CAD build for the part. Positions are in the model's coordinates, mm. Round coordinates to 2 decimals unless told otherwise and drop trailing zeros. Loops run counter-clockwise (first coordinate to the right, second up) from the corner with the lowest first, then second, coordinate; pieces in that order, holes last.
```python
from build123d import *

# Parameters (mm, degrees)
F0_W     = 101.6
F0_H     = 6.096
F1_DEPTH = 101.6
F2_W     = 6.35
F2_H     = 50.8
F2_H_2   = 25.4
F3_DEPTH = 25.4
F4_R     = 2.032


with BuildPart() as f1:
    # F0 (on Front) → F1 (new body)
    with BuildSketch(Plane.XZ):
        with Locations((2.470545, 16.174641)):
            Rectangle(F0_W, F0_H)
    extrude(amount=F1_DEPTH)

    # F2 (on face) → F3 (cut)
    with BuildSketch(Plane.XY.offset(19.222641)):
        with Locations((-45.154455, -50.8)):
            Rectangle(F2_W, F2_H)
        with Locations((50.095545, -12.7)):
            Rectangle(F2_W, F2_H_2)
        with Locations((50.095545, -88.9)):
            Rectangle(F2_W, F2_H_2)
    extrude(amount=-F3_DEPTH, mode=Mode.SUBTRACT)

    # F4
    f4_edges = [f1.edges().sort_by_distance(p)[0] for p in [
        (53.270545, -50.8, 19.222641),
        (46.920545, -88.9, 19.222641),
        (46.920545, -12.7, 19.222641),
        (53.270545, -50.8, 13.126641),
        (46.920545, -12.7, 13.126641),
        (46.920545, -88.9, 13.126641),
        (-41.979455, -50.8, 19.222641),
        (-48.329455, -12.7, 19.222641),
        (-48.329455, -88.9, 19.222641),
        (-41.979455, -50.8, 13.126641),
        (-48.329455, -12.7, 13.126641),
        (-48.329455, -88.9, 13.126641),
    ]]
    fillet(f4_edges, radius=F4_R)


solid = f1.part
```
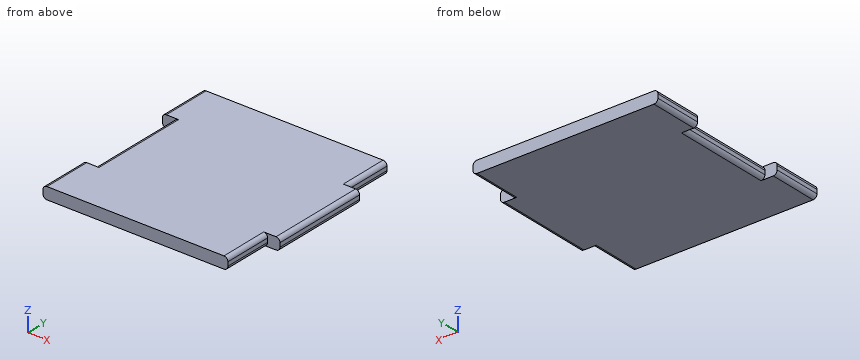
Item 1: Cut at A-A, the plane y = -63. Give the cut face in (x, z).
Answers follow:
outline: (-41.98, 15.16) arc R2.03 ccw to (-39.95, 13.13) - (51.24, 13.13) arc R2.03 ccw to (53.27, 15.16) - (53.27, 17.19) arc R2.03 ccw to (51.24, 19.22) - (-39.95, 19.22) arc R2.03 ccw to (-41.98, 17.19) - close
Item 2: Flat gauge pins, fed straight in: P1, Ø1.6, axis at y = -12, z = 16, coming from the +X side; P2, Ø0.6, axis at y = -44.5, z = 16.5, coming from the -X side. Where does each tip first touch, or does it go through?
Answers follow:
P1: stops at x = 46.92
P2: stops at x = -41.98
Item 3: Probe line 1 (X direction, y = -94, z = 17.25); line 2 (X direction, y = -34.5, z = 17.5). List the from-to ranges inside material, lowest first.
Answers follow:
line 1: x = -48.33 to 46.92
line 2: x = -41.96 to 53.25
